from build123d import *

# Parameters (mm, degrees)
SKETCH1_W               = 50
SKETCH1_H               = 110
BOSS_EXTRUDE1_DEPTH     = 2
SKETCH2_W               = 50
SKETCH2_H               = 110
SKETCH2_W_2             = 46
SKETCH2_H_2             = 106
BOSS_EXTRUDE3_DEPTH     = 11
SKETCH3_R               = 1.2
BOSS_EXTRUDE4_DEPTH     = 11
SKETCH4_W               = 52
SKETCH4_H               = 112
SKETCH4_W_2             = 50
SKETCH4_H_2             = 110
EXTRUDE_THIN1_DEPTH     = 13
FILLET2_R               = 2
EXTRUDE_THIN3_DEPTH     = 3
SKETCH6_R               = 1.8
BOSS_EXTRUDE5_DEPTH     = 2.8
SKETCH8_W               = 8
SKETCH8_H               = 3.6
CUT_EXTRUDE2_DEPTH      = 12.8
SKETCH11_W              = 13.1
SKETCH11_H              = 5.8
CUT_EXTRUDE5_DEPTH      = 3
SKETCH12_W              = 70
SKETCH12_H              = 9.973266712
CUT_EXTRUDE6_DEPTH      = 130
SKETCH13_W              = 46
SKETCH13_H              = 106
CUT_EXTRUDE7_DEPTH      = 130
SKETCH15_W              = 46
SKETCH15_H              = 106
BOSS_EXTRUDE6_DEPTH     = 60
SKETCH16_W              = 71.739839436
SKETCH16_H              = 55.166081701
CUT_EXTRUDE8_DEPTH      = 130
SKETCH17_W              = 110.8
SKETCH17_H              = 170.8
SKETCH17_W_2            = 48.4
SKETCH17_H_2            = 108.4
CUT_EXTRUDE_THIN1_DEPTH = 3
SKETCH18_W              = 3
SKETCH18_H              = 13.1
BOSS_EXTRUDE7_DEPTH     = 7
SKETCH19_W              = 3
SKETCH19_H              = 8
BOSS_EXTRUDE8_DEPTH     = 4.5
SKETCH20_R              = 6
SKETCH20_R_2            = 3
CUT_EXTRUDE9_DEPTH      = 4.5


with BuildPart() as part:
    # Sketch1 → Boss-Extrude1 (new body)
    with BuildSketch(Plane(origin=(0, 0, 0), x_dir=(1, 0, 0), z_dir=(0, 1, 0))):
        with Locations((-52.022587269, -1.919917864)):
            Rectangle(SKETCH1_W, SKETCH1_H)
    extrude(amount=BOSS_EXTRUDE1_DEPTH)

    # Sketch2 → Boss-Extrude3 (add)
    with BuildSketch(Plane(origin=(0, 2, 0), x_dir=(1, 0, 0), z_dir=(0, 1, 0))):
        with Locations((-52.022587269, -1.919917864)):
            Rectangle(SKETCH2_W, SKETCH2_H)
        with Locations((-52.022587269, -1.919917864)):
            Rectangle(SKETCH2_W_2, SKETCH2_H_2, mode=Mode.SUBTRACT)
    extrude(amount=BOSS_EXTRUDE3_DEPTH)

    # Sketch3 → Boss-Extrude4 (add)
    with BuildSketch(Plane(origin=(0, 2, 0), x_dir=(1, 0, 0), z_dir=(0, 1, 0))):
        with Locations((-31.022587269, 42.380082136)):
            Circle(SKETCH3_R)
        with Locations((-31.022587269, -52.919917864)):
            Circle(SKETCH3_R)
        with Locations((-56.322587269, 42.380082136)):
            Circle(SKETCH3_R)
        with Locations((-56.322587269, -52.919917864)):
            Circle(SKETCH3_R)
    extrude(amount=BOSS_EXTRUDE4_DEPTH)

    # Sketch4 → Extrude-Thin1 (add)
    with BuildSketch(Plane(origin=(0, 13, 0), x_dir=(1, 0, 0), z_dir=(0, 1, 0))):
        with Locations((-52.022587269, -1.919917864)):
            Rectangle(SKETCH4_W, SKETCH4_H)
        with Locations((-52.022587269, -1.919917864)):
            Rectangle(SKETCH4_W_2, SKETCH4_H_2, mode=Mode.SUBTRACT)
    extrude(amount=-EXTRUDE_THIN1_DEPTH)

    # Fillet2
    fillet2_edges = [part.edges().sort_by_distance(p)[0] for p in [
        (-26.022587269, 6.5, -54.080082136),
        (-26.022587269, 6.5, 57.919917864),
        (-78.022587269, 6.5, 57.919917864),
        (-78.022587269, 6.5, -54.080082136),
    ]]
    fillet(fillet2_edges, radius=FILLET2_R)

    # Sketch5 → Extrude-Thin3 (add)
    with BuildSketch(Plane(origin=(0, 13, 0), x_dir=(1, 0, 0), z_dir=(0, 1, 0))):
        with BuildLine():
            Line((-28.022587269, 54.080082136), (-76.022587269, 54.080082136))
            ThreePointArc((-76.022587269, 54.080082136), (-77.436800831, 53.494295698), (-78.022587269, 52.080082136))
            Line((-78.022587269, 52.080082136), (-78.022587269, -55.919917864))
            ThreePointArc((-78.022587269, -55.919917864), (-77.436800831, -57.334131427), (-76.022587269, -57.919917864))
            Line((-76.022587269, -57.919917864), (-28.022587269, -57.919917864))
            ThreePointArc((-28.022587269, -57.919917864), (-26.608373707, -57.334131427), (-26.022587269, -55.919917864))
            Line((-26.022587269, -55.919917864), (-26.022587269, 52.080082136))
            ThreePointArc((-26.022587269, 52.080082136), (-26.608373707, 53.494295698), (-28.022587269, 54.080082136))
        make_face()
        with BuildLine():
            Line((-28.022587269, 52.880082136), (-76.022587269, 52.880082136))
            ThreePointArc((-76.022587269, 52.880082136), (-76.588272694, 52.64576756), (-76.822587269, 52.080082136))
            Line((-76.822587269, 52.080082136), (-76.822587269, -55.919917864))
            ThreePointArc((-76.822587269, -55.919917864), (-76.588272694, -56.485603289), (-76.022587269, -56.719917864))
            Line((-76.022587269, -56.719917864), (-28.022587269, -56.719917864))
            ThreePointArc((-28.022587269, -56.719917864), (-27.456901844, -56.485603289), (-27.222587269, -55.919917864))
            Line((-27.222587269, -55.919917864), (-27.222587269, 52.080082136))
            ThreePointArc((-27.222587269, 52.080082136), (-27.456901844, 52.64576756), (-28.022587269, 52.880082136))
        make_face(mode=Mode.SUBTRACT)
    extrude(amount=EXTRUDE_THIN3_DEPTH)

    # Sketch6 → Boss-Extrude5 (add)
    with BuildSketch(Plane(origin=(0, 2, 0), x_dir=(1, 0, 0), z_dir=(0, 1, 0))):
        with Locations((-56.322587269, -52.919917864)):
            Circle(SKETCH6_R)
        with Locations((-31.022587269, -52.919917864)):
            Circle(SKETCH6_R)
        with Locations((-56.322587269, 42.380082136)):
            Circle(SKETCH6_R)
        with Locations((-31.022587269, 42.380082136)):
            Circle(SKETCH6_R)
    extrude(amount=BOSS_EXTRUDE5_DEPTH)

    # Sketch8 → Cut-Extrude2 (cut)
    with BuildSketch(Plane(origin=(-26.022587269, 0, 0), x_dir=(0, 0, -1), z_dir=(1, 0, 0))):
        with Locations((-44.619917864, 3.8)):
            Rectangle(SKETCH8_W, SKETCH8_H)
    extrude(amount=-CUT_EXTRUDE2_DEPTH, mode=Mode.SUBTRACT)

    # Sketch11 → Cut-Extrude5 (cut)
    with BuildSketch(Plane.ZY.offset(78.022587269)):
        with Locations((-43.530082136, 4.9)):
            Rectangle(SKETCH11_W, SKETCH11_H)
    extrude(amount=-CUT_EXTRUDE5_DEPTH, mode=Mode.SUBTRACT)

    # Sketch12 → Cut-Extrude6 (cut)
    with BuildSketch(Plane.XY.offset(57.919917864)):
        with Locations((-53.022587269, 15.377484965)):
            Rectangle(SKETCH12_W, SKETCH12_H)
    extrude(amount=-CUT_EXTRUDE6_DEPTH, mode=Mode.SUBTRACT)

    # Sketch13 → Cut-Extrude7 (cut)
    with BuildSketch(Plane(origin=(0, 2, 0), x_dir=(1, 0, 0), z_dir=(0, 1, 0))):
        with Locations((-52.022587269, -1.919917864)):
            Rectangle(SKETCH13_W, SKETCH13_H)
    extrude(amount=CUT_EXTRUDE7_DEPTH, mode=Mode.SUBTRACT)

    # Sketch15 → Boss-Extrude6 (add)
    with BuildSketch(Plane(origin=(0, 10.390851609, 0), x_dir=(1, 0, 0), z_dir=(0, 1, 0))):
        with BuildLine():
            Line((-76.022587269, -57.919917864), (-28.022587269, -57.919917864))
            ThreePointArc((-28.022587269, -57.919917864), (-26.608373707, -57.334131427), (-26.022587269, -55.919917864))
            Line((-26.022587269, -55.919917864), (-26.022587269, 52.080082136))
            ThreePointArc((-26.022587269, 52.080082136), (-26.608373707, 53.494295698), (-28.022587269, 54.080082136))
            Line((-28.022587269, 54.080082136), (-76.022587269, 54.080082136))
            ThreePointArc((-76.022587269, 54.080082136), (-77.436800831, 53.494295698), (-78.022587269, 52.080082136))
            Line((-78.022587269, 52.080082136), (-78.022587269, -55.919917864))
            ThreePointArc((-78.022587269, -55.919917864), (-77.436800831, -57.334131427), (-76.022587269, -57.919917864))
        make_face()
        with Locations((-52.022587269, -1.919917864)):
            Rectangle(SKETCH15_W, SKETCH15_H, mode=Mode.SUBTRACT)
    extrude(amount=BOSS_EXTRUDE6_DEPTH)

    # Sketch16 → Cut-Extrude8 (cut)
    with BuildSketch(Plane.XY.offset(57.919917864)):
        with Locations((-48.522353235, 51.583040851)):
            Rectangle(SKETCH16_W, SKETCH16_H)
    extrude(amount=-CUT_EXTRUDE8_DEPTH, mode=Mode.SUBTRACT)

    # Sketch17 → Cut-Extrude-Thin1 (cut)
    with BuildSketch(Plane(origin=(0, 24, 0), x_dir=(1, 0, 0), z_dir=(0, 1, 0))):
        with Locations((-52.022587269, -1.919917864)):
            Rectangle(SKETCH17_W, SKETCH17_H)
        with Locations((-52.022587269, -1.919917864)):
            Rectangle(SKETCH17_W_2, SKETCH17_H_2, mode=Mode.SUBTRACT)
    extrude(amount=-CUT_EXTRUDE_THIN1_DEPTH, mode=Mode.SUBTRACT)

    # Sketch18 → Boss-Extrude7 (add)
    with BuildSketch(Plane.XZ.offset(-7.8)):
        with Locations((-76.522587269, -43.530082136)):
            Rectangle(SKETCH18_W, SKETCH18_H)
    extrude(amount=BOSS_EXTRUDE7_DEPTH)

    # Sketch19 → Boss-Extrude8 (add)
    with BuildSketch(Plane.XZ.offset(-5.6)):
        with Locations((-27.522587269, 44.619917864)):
            Rectangle(SKETCH19_W, SKETCH19_H)
    extrude(amount=BOSS_EXTRUDE8_DEPTH)

    # Sketch20 → Cut-Extrude9 (cut)
    with BuildSketch(Plane(origin=(0, 2, 0), x_dir=(1, 0, 0), z_dir=(0, 1, 0))):
        with Locations((-65.022587269, -39.919917864)):
            Circle(SKETCH20_R)
        with Locations((-65.022587269, 36.080082136)):
            Circle(SKETCH20_R_2)
    extrude(amount=-CUT_EXTRUDE9_DEPTH, mode=Mode.SUBTRACT)


solid = part.part
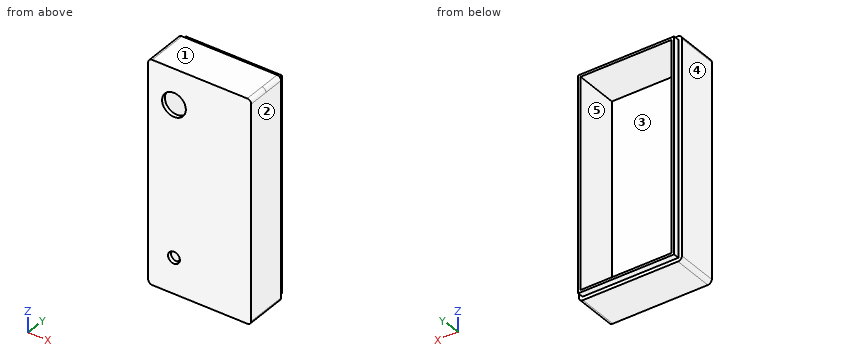
Model file for the job. Use its own axes, mm. Face numbers are marked on the shaded views. A direction names the side the tool comes from. Coordinates: 2 decimals unless noted, no trailing zeros. Write each loop counter-clockwise with the first axis right and the second up, starting at its lowest first coordinate (ties: lowest second). Pieces come first, ordered by that corner, then holes. Notation, with made-up numbers: (5.25, 51) - (52.25, 51) arc R20 cw to (52.25, 59) - close; hole circle Ø7 at (41, -24). An arc over 180 degrees is marked (long way). Write each question's results on one line, items separated by ' | '. Start each with the question number.
1) Cut at C-C (x = -63.5). Write the cut outline in (y, z).
2) Flat gauge pins, fed straight in: P1, Ø0.9, axis at y = 22.5, z = -4, coming from the -X side; P2, Ø5.5, axis at x = -65.02, z = -36.08, coming from the +Y side; P3, Ø3, axis at x = -45.5, z = 13, coming from the +Y side; P4, Ø2.5, axis at x = -53.5, y = 23, coming from the -Z side. Where does each tip first touch, or does it go through?
3) Mould opens along Z. For the marked faces 1, 2 and 3 say: pulls with the +Z half, pulls with the -Z half, needs draft (parallel to the pull), parting line crosses it, or undercut.
4) Cut at A-A (y = 22.5). Write the cut outline in (x, z), then the cut area to 3 significant figures.
5) 3-axis set-ups, long thin cutter, end or side, ignore diameter. For the marked faces 4 and 5: which of +Z, -Z, +X, -X, +Y, -Y reach the whole face in a straight line?
6) Cut at B-B (z = 20.5). Write the cut outline in (x, y), then the cut area to 3 significant figures.
7) Cut at D-D (x = -44). Write the cut outline in (y, z).
8) Probe line 1 along X through (y, z) = (4, 1); line 2 along Z through (x, y) = (-38, 6.5); line 3 along Z through (x, y) = (-33, 22.75). List the from-to ranges inside material, lowest first. Write a range as from..to.
Returned:
1) outline: (0, -54.08) - (21, -54.08) - (21, -52.28) - (24, -52.28) - (24, -51.08) - (2, -51.08) - (2, -38.66) - (0, -38.66) - close; (0, -33.5) - (2, -33.5) - (2, 34.12) - (0, 34.12) - close; (0, 45.72) - (2, 45.72) - (2, 54.92) - (24, 54.92) - (24, 56.12) - (21, 56.12) - (21, 57.92) - (0, 57.92) - close
2) P1: x = -76.22 | P2: through | P3: y = 2 | P4: z = -52.28
3) face 1: pulls with the +Z half | face 2: needs draft | face 3: undercut
4) outline: (-76.22, -52.28) - (-27.82, -52.28) - (-27.82, 56.12) - (-76.22, 56.12) - close; hole (-75.02, -51.08) - (-29.02, -51.08) - (-29.02, 54.92) - (-75.02, 54.92) - close | area: 371 mm^2
5) face 4: +Z, -Z, -X, +Y, -Y | face 5: +Y
6) outline: (-78.02, 0) - (-26.02, 0) - (-26.02, 21) - (-27.82, 21) - (-27.82, 24) - (-29.02, 24) - (-29.02, 2) - (-75.02, 2) - (-75.02, 24) - (-76.22, 24) - (-76.22, 21) - (-78.02, 21) - close | area: 225 mm^2
7) outline: (0, -54.08) - (21, -54.08) - (21, -52.28) - (24, -52.28) - (24, -51.08) - (2, -51.08) - (2, 54.92) - (24, 54.92) - (24, 56.12) - (21, 56.12) - (21, 57.92) - (0, 57.92) - close
8) line 1: -78.02..-75.02, -29.02..-26.02 | line 2: -54.08..-51.08, 54.92..57.92 | line 3: -52.28..-51.08, 54.92..56.12
